from build123d import *

# Parameters (mm, degrees)
F1_DEPTH = 319.024


with BuildPart() as f1:
    # F0 (on Top) → F1 (new body)
    with BuildSketch(Plane.XY):
        with BuildLine():
            Line((-3.723805, 0), (0, 0))
            Line((0, 0), (38.15455, 0))
            Line((38.15455, 0), (38.15455, 7.313689))
            Line((38.15455, 7.313689), (32.867547, 7.313689))
            ThreePointArc((32.867547, 7.313689), (25.972411, 3.959021), (19.077275, 7.313689))
            Line((19.077275, 7.313689), (14.36303, 7.313689))
            ThreePointArc((14.36303, 7.313689), (7.181515, 3.352431), (0, 7.313689))
            Line((0, 7.313689), (-3.723805, 7.313689))
            Line((-3.723805, 7.313689), (-3.723805, 0))
        make_face()
    extrude(amount=F1_DEPTH)


solid = f1.part
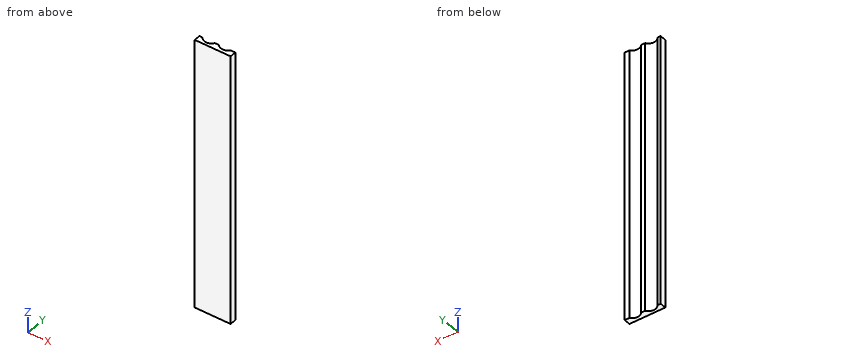
Here's how the part is built. I have some questions about the finished solid (model axes, mm). Round coordinates to 2 decimals unless told otherwise and drop trailing zeros. Write each loop counter-clockwise with the first axis right and the second up, starting at its lowest first coordinate (ties: lowest second). Pieces come first, ordered by that corner, then holes.
1. Will this pin go through, and if not, where does the flat tip stop? pin 1 Ø1 at (x, z) = (13, 178) entering from +Y.
2. I need wall thicknesses on L1, parallel to X at y = 5, z = 149.5; L2, parallel to X at y = 6.5, z = 133.5; L3, parallel to Y at x = 26.5, z = 216. Which ranges of each line are inside material? Lowest first, please.
3. Suppose I cut it at B-B (z = 36). List the corners of the cut face in (x, y) for me.
4. Suppose I cut it at A-A (y = 6). List the corners of the cut face in (x, z) for me.
Answer sheet:
1. pin 1: stops at y = 6.17
2. L1: x = -3.72 to 2.16, 12.21 to 21.83, 30.12 to 38.15
2. L2: x = -3.72 to 0.58, 13.78 to 19.8, 32.14 to 38.15
2. L3: y = 0 to 3.97
3. outline: (-3.72, 0) - (38.15, 0) - (38.15, 7.31) - (32.87, 7.31) arc R8.76 cw to (19.08, 7.31) - (14.36, 7.31) arc R8.49 cw to (0, 7.31) - (-3.72, 7.31) - close
4. outline: (-3.72, 0) - (1.02, 0) - (1.02, 319.02) - (-3.72, 319.02) - close; (13.34, 0) - (20.35, 0) - (20.35, 319.02) - (13.34, 319.02) - close; (31.59, 0) - (38.15, 0) - (38.15, 319.02) - (31.59, 319.02) - close
